Geometry: final body of the model. Coordinates: model frame, mm. Round coordinates to 2 decimals unless told otherwise and drop trailing zeros. Loops run counter-clockwise (first coordinate to the right, second up) from the corner with the lowest first, then second, coordinate; pieces in that order, holes last. Notation, with made-up numbers: M 6,68 L 35,68 A25 cw 35,91 Z; hole C -9,-9.5 d10. An arc over 180 degrees is marked long. Return JSON: item names as keys, results as strings.
from build123d import *

# Parameters (mm, degrees)
SKETCH1_W           = 90
SKETCH1_H           = 20
SKETCH1_R           = 7.95
SKETCH1_R_2         = 8
SKETCH1_R_3         = 8.025
SKETCH1_R_4         = 8.05
BOSS_EXTRUDE1_DEPTH = 3.175
FILLET1_R           = 10


with BuildPart() as part:
    # Sketch1 → Boss-Extrude1 (new body)
    with BuildSketch(Plane(origin=(0, 0, 0), x_dir=(1, 0, 0), z_dir=(0, 1, 0))):
        Rectangle(SKETCH1_W, SKETCH1_H)
        with Locations(Location((-30, 0, 0), (0, 0, 270))):
            Circle(SKETCH1_R, mode=Mode.SUBTRACT)
        with Locations(Location((-10, 0, 0), (0, 0, 270))):
            Circle(SKETCH1_R_2, mode=Mode.SUBTRACT)
        with Locations(Location((10, 0, 0), (0, 0, 270))):
            Circle(SKETCH1_R_3, mode=Mode.SUBTRACT)
        with Locations(Location((30, 0, 0), (0, 0, 270))):
            Circle(SKETCH1_R_4, mode=Mode.SUBTRACT)
    extrude(amount=BOSS_EXTRUDE1_DEPTH)

    # Fillet1
    fillet1_edges = [part.edges().sort_by_distance(p)[0] for p in [
        (-45, 1.5875, -10),
        (-45, 1.5875, 10),
    ]]
    fillet(fillet1_edges, radius=FILLET1_R - 0.0001)  # a hair under: the kernel refuses the full size


solid = part.part
Q1. Pin query (flat end, axial travel): pin 1 (10 mm diameter, centred on x = -30.5, z = -5, fed in from -Y). Return the tip coordinate at first contact, or that it passes through.
Determined:
{"pin 1": "stops at y = 0"}
Q2. Section query B-B (y = 0.65). State how many separate pieces and enclosed holes the cut face has, plus the area to 3 significant figures.
Determined:
{"separate pieces": "1", "enclosed holes": "4", "area": "952 mm^2"}
Q3. Section query C-C (z = -3.5). Output: boundary loops of the cut face in (x, y) (3 decimals).
Determined:
{"outline": "M -44.368,0 L -37.138,0 L -37.138,3.175 L -44.368,3.175 Z; M -22.862,0 L -17.194,0 L -17.194,3.175 L -22.862,3.175 Z; M -2.806,0 L 2.778,0 L 2.778,3.175 L -2.806,3.175 Z; M 17.222,0 L 22.751,0 L 22.751,3.175 L 17.222,3.175 Z; M 37.249,0 L 45,0 L 45,3.175 L 37.249,3.175 Z"}
Q4. Material intervals for L1, parallel to X at y = 2.3, z = 0 (3 decimals); L2, parallel to Z at x = -9.5, y = 1.4; L3, parallel to Z at x = -9, y = 0.85, sorted ascending.
Determined:
{"L1": "x = -45 to -37.95, -22.05 to -18, -2 to 1.975, 18.025 to 21.95, 38.05 to 45", "L2": "z = -10 to -7.98, 7.98 to 10", "L3": "z = -10 to -7.94, 7.94 to 10"}
Q5. Pull-direction query (X, two-part tool) for faces 1 (the cylindrical face through (-22.118, 1.565, -1.035)), 2 (the cylindrical face through (-42.15, 1.61, -6.99)), 3 (the flat face through (-1, 0, 0)); classes: pulls with the +X half, pulls with the -X half, needs draft (parallel to the pull), parting line crosses it, or undercut.
Determined:
{"face 1": "undercut", "face 2": "pulls with the -X half", "face 3": "needs draft"}
Q6. Section query A-A (x = -30). Output: boundary loops of the cut face in (y, z) (3 decimals), plus the area to 3 significant figures.
Determined:
{"outline": "M 0,-10 L 3.175,-10 L 3.175,-7.95 L 0,-7.95 Z; M 0,7.95 L 3.175,7.95 L 3.175,10 L 0,10 Z", "area": "13.0 mm^2"}
Q7. Section query D-D (x = -10). Output: boundary loops of the cut face in (y, z) (3 decimals).
Determined:
{"outline": "M 0,-10 L 3.175,-10 L 3.175,-8 L 0,-8 Z; M 0,8 L 3.175,8 L 3.175,10 L 0,10 Z"}
